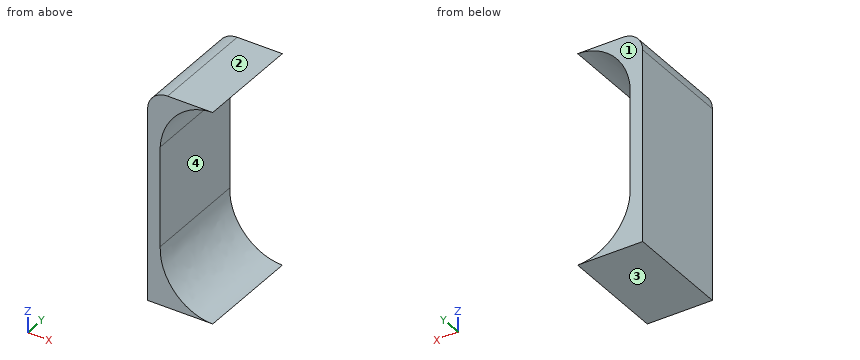
```python
from build123d import *

# Parameters (mm, degrees)
SKETCH1_W           = 60
SKETCH1_H           = 80
BOSS_EXTRUDE1_DEPTH = 160
CUT_EXTRUDE1_DEPTH  = 182.383571472
FILLET1_R           = 15


with BuildPart() as part:
    # Sketch1 → Boss-Extrude1 (new body)
    with BuildSketch(Plane.XY):
        Rectangle(SKETCH1_W, SKETCH1_H)
    extrude(amount=BOSS_EXTRUDE1_DEPTH)

    # Sketch2 → Cut-Extrude1 (cut, through all)
    with BuildSketch(Plane(origin=(0, 40, 0), x_dir=(1, 0, 0), z_dir=(0, 1, 0))):
        with BuildLine():
            Line((-20.538426818, -44.05376626), (-20.538426818, -80))
            Line((-20.538426818, -80), (30, -80))
            Line((30, -80), (30, 0))
            Line((30, 0), (19, 0))
            add(Edge.make_bspline(
                [(19, 0), (-4.370713607, -0.406174328), (-21.495622782, -22.117426015), (-20.538426818, -44.05376626)],
                knots=[0, 0, 0, 0, 1, 1, 1, 1], degree=3))
        make_face()
        with BuildLine():
            Line((-20.538426818, -80), (-20.538426818, -115.94623374))
            Line((-20.538426818, -115.94623374), (-20.538426818, -119.465924684))
            add(Edge.make_bspline(
                [(19, -160), (-3.118929784, -159.61558121), (-19.643213017, -140.147251157), (-20.538426818, -119.465924684)],
                knots=[0, 0, 0, 0, 0.946437929, 0.946437929, 0.946437929, 0.946437929], degree=3))
            Line((19, -160), (30, -160))
            Line((30, -160), (30, -80))
            Line((30, -80), (-20.538426818, -80))
        make_face()
    extrude(amount=-CUT_EXTRUDE1_DEPTH, mode=Mode.SUBTRACT)

    # Fillet1
    fillet1_edges = [part.edges().sort_by_distance(p)[0] for p in [
        (-30, 0, 160),
    ]]
    fillet(fillet1_edges, radius=FILLET1_R)


solid = part.part
```
Can you work these out from the model? Positions are in its coordinate system, mm. Face numbers are marked on the shaded views. Coordinates: 2 decimals unless noted, no trailing zeros. Order: outer loops, then holes, each group sorted by start corner. A loop starts at its lowest first (then second) coordinate and runs counter-clockwise, first axis right, second up.
1. I need wall thicknesses on line 1 (Z direction, x = -5, y = -31.5); line 2 (Z direction, x = -14.5, y = 20.5); line 3 (X direction, y = -0.5, z = 46.5). Which ranges of each line are inside material? Lowest first, please.
2. If we section it at A-A (z = 112): Please give me the cut outline in (x, y), then the cut area to 3 significant figures.
3. I'm going to push flat-ended pins straight in: pin 1 (1.5 mm diameter, centred on y = 21, z = 127.5, fed in from +X); pin 2 (1 mm diameter, centred on x = -18, z = 31.5, fed in from -Y). Where does each tip first touch, or does it pass through?
4. Thinking about a two-plate mould opening in Z: for the marked faces 1, 2, 3 and 4, which applies, +Z half, -Z half, draft (parallel to the pull), parting line (faces both ways), or undercut?
Entries:
1. line 1: z = 0 to 9.12, 150.88 to 160
1. line 2: z = 0 to 20.39, 139.61 to 160
1. line 3: x = -30 to -20.54
2. outline: (-30, -40) - (-20.54, -40) - (-20.54, 40) - (-30, 40) - close
2. area: 757 mm2
3. pin 1: stops at x = -19.21
3. pin 2: passes through
4. face 1: draft
4. face 2: +Z half
4. face 3: -Z half
4. face 4: undercut
